The listing builds one solid part. Answer for the finished solid, in the listing's coordinates (mm). A direction names the side the tool comes from. Coordinates: 2 decimals unless noted, no trailing zeros. Loops run counter-clockwise (first coordinate to the right, second up) from the corner with the lowest first, then second, coordinate; pieces in that order, holes last. Notation, with made-up numbers: (-40, -20.5) - (-32, -20.5) arc R25 cw to (-32, -4.5) - close; hole circle Ø6 at (67.5, 41.25). An arc over 180 degrees is marked (long way). Return JSON: item names as keys, results as strings. Group by question number.
1. Each of these flat-tipped pins is pushed along its axis until it touches: P1, Ø1.6, axis at x = 9, y = -14, coming from the +Z side; P2, Ø0.8, axis at x = 11.5, y = 2, coming from the +Z side; P3, Ø0.6, axis at x = 8.5, z = 1.5, coming from the +Y side. Where does it stop, or does it pass through?
2. Section B-B (y = -6) is taken. Write down the section's boundary in (x, z), and give its area (3 significant figures).
3. Find the intervals of material crossed by line 1 along X through (y, z) = (3.5, 1.6); line 2 along Y through (x, z) = (5, 1.65); line 3 along Y through (x, z) = (1.75, 1.4), in increasing order.
4. The mould has two halves that part along X. Classify faces 5 (the face through (3, 1, 1.5)), 6 (the face through (7, -14, 1)), 7 (the face through (17.03, 1, 1)), 8 (the face through (-2.97, 1, 1)): pulls with the +X half, pulls with the -X half, needs draft (parallel to the pull), parting line crosses it, or undercut.
5. Which of the six approach directions +Z, -Z, +X, -X, +Y, -Y give full straight-line access (tool end or side, diameter ignored) to faces 1 (the face through (12, 1, 1.5)), 2 (the face through (7, 15, 1)), 3 (the face through (6.9, -12.677, 1.5)), 4 (the face through (7, 1, 0))?
6. Section A-A (x = 10) is taken. Write down the section's boundary in (y, z), and give its area (3 significant figures).
7. Section C-C (x = 2.5) is taken. Write down the section's boundary in (y, z).
```python
from build123d import *

# Parameters (mm, degrees)
F0_W     = 20
F0_H     = 31
F1_DEPTH = 1
F2_W     = 20
F2_H     = 27
F3_DEPTH = 1
F4_W     = 1.5
F4_H     = 17
F5_DEPTH = 0.5


with BuildPart() as f1:
    # F0 (on Top) → F1 (new body)
    with BuildSketch(Plane.XY):
        with Locations((7.02957, 0.822581)):
            Rectangle(F0_W, F0_H)
    extrude(amount=F1_DEPTH)

    # F2 (on face) → F3 (join)
    with BuildSketch(Plane.XY.offset(1)):
        with Locations((7.02957, 0.822581)):
            Rectangle(F2_W, F2_H)
    extrude(amount=F3_DEPTH)

    # F4 (on face) → F5 (cut)
    with BuildSketch(Plane.XY.offset(2)):
        with Locations((2.52957, 0.822581)):
            Rectangle(F4_W, F4_H)
        with Locations((5.52957, 0.822581)):
            Rectangle(F4_W, F4_H)
        with Locations((8.52957, 0.822581)):
            Rectangle(F4_W, F4_H)
        with Locations((11.52957, 0.822581)):
            Rectangle(F4_W, F4_H)
    extrude(amount=-F5_DEPTH, mode=Mode.SUBTRACT)


solid = f1.part
```
The answers:
{
 "1": {"P1": "stops at z = 1", "P2": "stops at z = 1.5", "P3": "stops at y = 14.32"},
 "2": {"outline": "(-2.97, 0) - (17.03, 0) - (17.03, 2) - (12.28, 2) - (12.28, 1.5) - (10.78, 1.5) - (10.78, 2) - (9.28, 2) - (9.28, 1.5) - (7.78, 1.5) - (7.78, 2) - (6.28, 2) - (6.28, 1.5) - (4.78, 1.5) - (4.78, 2) - (3.28, 2) - (3.28, 1.5) - (1.78, 1.5) - (1.78, 2) - (-2.97, 2) - close", "area": "37.0 mm2"},
 "3": {"line 1": "x = -2.97 to 1.78, 3.28 to 4.78, 6.28 to 7.78, 9.28 to 10.78, 12.28 to 17.03", "line 2": "y = -12.68 to -7.68, 9.32 to 14.32", "line 3": "y = -12.68 to 14.32"},
 "4": {"face 5": "undercut", "face 6": "needs draft", "face 7": "pulls with the +X half", "face 8": "pulls with the -X half"},
 "5": {"face 1": "+Z", "face 2": "+Z, +X, -X, +Y", "face 3": "+Z, +X, -X, -Y", "face 4": "-Z, +X, -X, +Y, -Y"},
 "6": {"outline": "(-14.68, 0) - (16.32, 0) - (16.32, 1) - (14.32, 1) - (14.32, 2) - (-12.68, 2) - (-12.68, 1) - (-14.68, 1) - close", "area": "58.0 mm2"},
 "7": {"outline": "(-14.68, 0) - (16.32, 0) - (16.32, 1) - (14.32, 1) - (14.32, 2) - (9.32, 2) - (9.32, 1.5) - (-7.68, 1.5) - (-7.68, 2) - (-12.68, 2) - (-12.68, 1) - (-14.68, 1) - close"}
}
